from build123d import *

# Parameters (mm, degrees)
SKIZZE1_W                          = 15
SKIZZE1_H                          = 15
AUFSATZ_LINEAR_AUSTRAGEN1_DEPTH    = 10
FASE1_SIZE                         = 1
SKIZZE1_2_W                        = 15
SKIZZE1_2_H                        = 15
AUFSATZ_LINEAR_AUSTRAGEN2_DEPTH    = 2
VERRUNDUNG1_R                      = 1
SKIZZE2_W                          = 24
SKIZZE2_H                          = 12
AUFSATZ_LINEAR_AUSTRAGEN3_DEPTH    = 24
F_1_0_1_DURCHMESSER_BOHRUNG1_D     = 1
F_1_0_1_DURCHMESSER_BOHRUNG1_DEPTH = 12
F_1_0_1_DURCHMESSER_BOHRUNG1_TIP   = 0.30043031
F_1_0_1_DURCHMESSER_BOHRUNG2_D     = 1
F_1_0_1_DURCHMESSER_BOHRUNG2_DEPTH = 2.2
F_1_0_1_DURCHMESSER_BOHRUNG2_TIP   = 0.30043031
F_3_0_3_DURCHMESSER_BOHRUNG1_D     = 3
F_3_0_3_DURCHMESSER_BOHRUNG1_DEPTH = 9
F_3_0_3_DURCHMESSER_BOHRUNG1_TIP   = 0.901290929
F_2_0_2_DURCHMESSER_BOHRUNG1_D     = 2
F_2_0_2_DURCHMESSER_BOHRUNG1_DEPTH = 1
F_2_0_2_DURCHMESSER_BOHRUNG1_TIP   = 0.600860619
VERRUNDUNG6_R                      = 0.3


with BuildPart() as part:
    # Skizze1 → Aufsatz-Linear austragen1 (new body)
    with BuildSketch(Plane.XY):
        Rectangle(SKIZZE1_W, SKIZZE1_H)
        with BuildLine():
            Line((-5.1, 0), (5.1, 0))
            ThreePointArc((5.1, 0), (0, 5.1), (-5.1, 0))
        make_face(mode=Mode.SUBTRACT)
    extrude(amount=AUFSATZ_LINEAR_AUSTRAGEN1_DEPTH)

    # Fase1
    fase1_edges = [part.edges().sort_by_distance(p)[0] for p in [
        (0, 5.1, 10),
        (0, 0, 10),
    ]]
    chamfer(fase1_edges, length=FASE1_SIZE)

    # Skizze1_2 → Aufsatz-Linear austragen2 (add)
    with BuildSketch(Plane.XY):
        Rectangle(SKIZZE1_2_W, SKIZZE1_2_H)
        with BuildLine():
            ThreePointArc((5.1, 0), (0, 5.1), (-5.1, 0))
            Line((-5.1, 0), (5.1, 0))
        make_face(mode=Mode.SUBTRACT)
        with BuildLine():
            Line((-5.1, 0), (5.1, 0))
            ThreePointArc((5.1, 0), (0, 5.1), (-5.1, 0))
        make_face()
    extrude(amount=-AUFSATZ_LINEAR_AUSTRAGEN2_DEPTH)

    # Verrundung1
    verrundung1_edges = [part.edges().sort_by_distance(p)[0] for p in [
        (-7.5, 0, 10),
        (0, -7.5, 10),
        (7.5, 0, 10),
        (0, 7.5, 10),
        (7.5, -7.5, 4),
        (-7.5, -7.5, 4),
        (-7.5, 7.5, 4),
        (7.5, 7.5, 4),
    ]]
    fillet(verrundung1_edges, radius=VERRUNDUNG1_R)

    # Skizze2 → Aufsatz-Linear austragen3 (add)
    with BuildSketch(Plane(origin=(0, 0, -2), x_dir=(-1, 0, 0), z_dir=(0, 0, -1))):
        Rectangle(SKIZZE2_W, SKIZZE2_H)
    extrude(amount=AUFSATZ_LINEAR_AUSTRAGEN3_DEPTH)

    # Skizze12 → Schnitt-Rotation1 (revolve, cut)
    with BuildSketch(Plane(origin=(0, 0, 0), x_dir=(1, 0, 0), z_dir=(0, 1, 0)), mode=Mode.PRIVATE) as schnitt_rotation1_sk:
        Polygon((-1, 2), (-4.879193576, 24), (0, 24), (0, 2), align=None)
    revolve(schnitt_rotation1_sk.sketch.rotate(Axis((0, 0, -2), (0, 0, -1)), 180), axis=Axis((0, 0, -2), (0, 0, -1)), mode=Mode.SUBTRACT)  # turned: the seam where the file's is

    # 1.0 _1_ Durchmesser Bohrung1
    with Locations(Plane(origin=(12, 0, -12), x_dir=(0, 0, 1), z_dir=(1, 0, 0))):
        with Locations((8, -1.3)):
            Hole(F_1_0_1_DURCHMESSER_BOHRUNG1_D / 2, depth=F_1_0_1_DURCHMESSER_BOHRUNG1_DEPTH)
            with Locations((0, 0, -(F_1_0_1_DURCHMESSER_BOHRUNG1_DEPTH + F_1_0_1_DURCHMESSER_BOHRUNG1_TIP / 2))):  # 118° drill point
                Cone(0, F_1_0_1_DURCHMESSER_BOHRUNG1_D / 2, F_1_0_1_DURCHMESSER_BOHRUNG1_TIP, mode=Mode.SUBTRACT)

    # 1.0 _1_ Durchmesser Bohrung2
    with Locations(Plane(origin=(0, 0, -26), x_dir=(-1, 0, 0), z_dir=(0, 0, -1))):
        with Locations((0, 4.170639233)):
            Hole(F_1_0_1_DURCHMESSER_BOHRUNG2_D / 2, depth=F_1_0_1_DURCHMESSER_BOHRUNG2_DEPTH)
            with Locations((0, 0, -(F_1_0_1_DURCHMESSER_BOHRUNG2_DEPTH + F_1_0_1_DURCHMESSER_BOHRUNG2_TIP / 2))):  # 118° drill point
                Cone(0, F_1_0_1_DURCHMESSER_BOHRUNG2_D / 2, F_1_0_1_DURCHMESSER_BOHRUNG2_TIP, mode=Mode.SUBTRACT)

    # 3.0 _3_ Durchmesser Bohrung1
    with Locations(Plane(origin=(12, 0, -12), x_dir=(0, 0, 1), z_dir=(1, 0, 0))):
        with Locations((8, -1.3)):
            Hole(F_3_0_3_DURCHMESSER_BOHRUNG1_D / 2, depth=F_3_0_3_DURCHMESSER_BOHRUNG1_DEPTH)
            with Locations((0, 0, -(F_3_0_3_DURCHMESSER_BOHRUNG1_DEPTH + F_3_0_3_DURCHMESSER_BOHRUNG1_TIP / 2))):  # 118° drill point
                Cone(0, F_3_0_3_DURCHMESSER_BOHRUNG1_D / 2, F_3_0_3_DURCHMESSER_BOHRUNG1_TIP, mode=Mode.SUBTRACT)

    # 2.0 _2_ Durchmesser Bohrung1
    with Locations(Plane(origin=(0, 0, -26), x_dir=(-1, 0, 0), z_dir=(0, 0, -1))):
        with Locations((0, 4.170639233)):
            Hole(F_2_0_2_DURCHMESSER_BOHRUNG1_D / 2, depth=F_2_0_2_DURCHMESSER_BOHRUNG1_DEPTH)
            with Locations((0, 0, -(F_2_0_2_DURCHMESSER_BOHRUNG1_DEPTH + F_2_0_2_DURCHMESSER_BOHRUNG1_TIP / 2))):  # 118° drill point
                Cone(0, F_2_0_2_DURCHMESSER_BOHRUNG1_D / 2, F_2_0_2_DURCHMESSER_BOHRUNG1_TIP, mode=Mode.SUBTRACT)

    # Verrundung6
    verrundung6_edges = [part.edges().sort_by_distance(p)[0] for p in [
        (-12, 0, -2),
        (-12, -6, -14),
        (-9.75, 6, -2),
        (9.75, 6, -2),
        (-12, 6, -14),
        (12, 0, -2),
        (12, 6, -14),
        (9.75, -6, -2),
        (-9.75, -6, -2),
        (12, -6, -14),
        (-12, 0, -26),
        (0, 6, -26),
        (12, 0, -26),
        (0, -6, -26),
    ]]
    fillet(verrundung6_edges, radius=VERRUNDUNG6_R)


solid = part.part
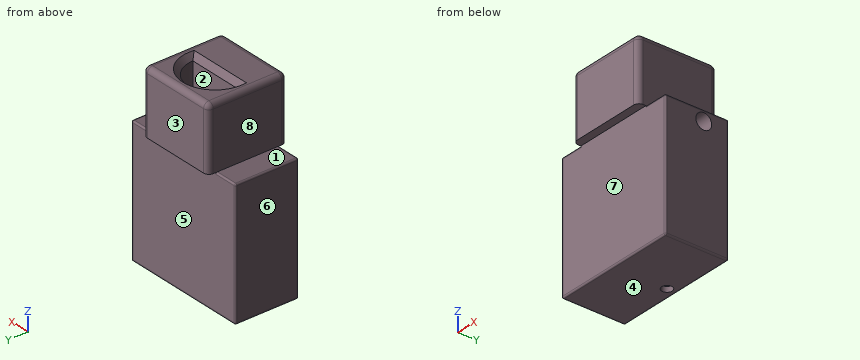
Build history of the part. All positions in model axes, mm. Face numbers are marked on the shaded views. A direction names the side the tool comes from. Round coordinates to 2 decimals unless told otherwise and drop trailing zeros. Write each loop counter-clockwise with the first axis right and the second up, starting at its lowest first coordinate (ties: lowest second). Pieces come first, ordered by that corner, then holes. Notation, with made-up numbers: M 21.25,37.25 L 32.25,37.25 A13 cw 32.25,42.25 Z; hole C -3.75,-8 d11. An arc over 180 degrees is marked long. Answer in a Markdown table with one row per item.
1. Probe L1, parallel to Y at x = 1.95, z = -4; L2, parallel to Y at x = 0, z = -24.2; L3, parallel to Y at x = 1.2, z = -4. List the from-to ranges inside material, lowest first. Write a range as [from, to].
Geometry check:
| item | result |
|---|---|
| L1 | [-6, 0.8], [1.8, 6] |
| L2 | [-6, 3.67], [4.67, 6] |
| L3 | [-6, -0.62], [0.62, 0.8], [1.8, 6] |
2. Saw through at A-A (x = -10.5). List the corners of the cut face in (y, z).
Geometry check:
| item | result |
|---|---|
| outline | M -6,-25.7 A0.3 ccw -5.7,-26 L 5.7,-26 A0.3 ccw 6,-25.7 L 6,-2.3 A0.3 ccw 5.7,-2 L -5.7,-2 A0.3 ccw -6,-2.3 Z |
3. Which spindle directions (+Z, -Z, +X, -X, +Y, -Y) get a long thin tool onto all of the face, cutting with end or side? Do the marked faces 4, 5, 6, 7 and 8. Say none if no direction does.
Geometry check:
| item | result |
|---|---|
| face 4 | -Z, +X, -X, +Y, -Y |
| face 5 | -Z, +X, -X, +Y |
| face 6 | +Z, -Z, -X, +Y, -Y |
| face 7 | -Z, +X, -X, -Y |
| face 8 | +Z, -X, +Y, -Y |
4. Saw through at B-B (z = -12). List the corners of the cut face in (x, y).
Geometry check:
| item | result |
|---|---|
| outline | M -12,-5.7 A0.3 ccw -11.7,-6 L 11.7,-6 A0.3 ccw 12,-5.7 L 12,5.7 A0.3 ccw 11.7,6 L -11.7,6 A0.3 ccw -12,5.7 Z; hole C 0,0 d5.53 |
5. Mould opens along Y. For the marked faces 1, 2 and 3 say: +Y half, -Y half, draft (parallel to the pull), parting line (faces both ways), or undercut.
Geometry check:
| item | result |
|---|---|
| face 1 | draft |
| face 2 | undercut |
| face 3 | +Y half |
6. Flat gauge pins, fed straight in: P1, Ø5.5, axis at y = 2, z = 6, coming from the +X side; P2, Ø4.5, axis at x = -9, y = 1, coming from the +Z side; P3, Ø4.5, axis at x = 10, y = -2, coming from the +Z side. Where does each tip first touch, or does it go through?
Geometry check:
| item | result |
|---|---|
| P1 | x = 7.5 |
| P2 | z = 9.97 |
| P3 | z = -2 |
7. Saw through at C-C (z = -21). List the corners of the cut face in (x, y), and give its area (3 significant figures).
Geometry check:
| item | result |
|---|---|
| outline | M -12,-5.7 A0.3 ccw -11.7,-6 L 11.7,-6 A0.3 ccw 12,-5.7 L 12,5.7 A0.3 ccw 11.7,6 L -11.7,6 A0.3 ccw -12,5.7 Z; hole C 0,0 d8.7 |
| area | 228 mm2 |
